Geometry check sheet. Reference: the model listing, model coordinates, mm. Face numbers are marked on the shaded views. A direction names the side the tool comes from. Round coordinates to 2 decimals unless told otherwise and drop trailing zeros. Write each loop counter-clockwise with the first axis right and the second up, starting at its lowest first coordinate (ties: lowest second). Pieces come first, ordered by that corner, then holes. Notation, with made-up numbers: (-9, 41.5) -> (29, 41.5) arc R22 ccw to (29, 48.5) -> close; hole circle Ø9 at (79, -23). An arc over 180 degrees is marked (long way). Return JSON: item names as keys, results as strings. Group by question number.
from build123d import *

# Parameters (mm, degrees)
EXTRUDE_1_DEPTH     = 3
SKETCH_2_R          = 1.6
CUT_EXTRUDE_1_DEPTH = 3


with BuildPart() as part:
    # 草图1 → 凸台-拉伸1 (new body)
    with BuildSketch(Plane.XY):
        Polygon((0, 48), (0, 0), (20, 0), (49.052558883, 16.773502692), (39.052558883, 34.094010768), (20, 23.094010768), (20, 48), align=None)
    extrude(amount=EXTRUDE_1_DEPTH)

    # 草图2 → 切除-拉伸1 (cut)
    with BuildSketch(Plane(origin=(0, 0, 0), x_dir=(-1, 0, 0), z_dir=(0, 0, -1))):
        with Locations((-42.222431864, 18.603629711)):
            Circle(SKETCH_2_R)
        with Locations((-37.222431864, 27.263883749)):
            Circle(SKETCH_2_R)
        with Locations((-26.830127019, 21.263883749)):
            Circle(SKETCH_2_R)
        with Locations((-31.830127019, 12.603629711)):
            Circle(SKETCH_2_R)
        with Locations((-16, 7)):
            Circle(SKETCH_2_R)
        with Locations((-16, 17)):
            Circle(SKETCH_2_R)
        with Locations((-4, 7)):
            Circle(SKETCH_2_R)
        with Locations((-4, 17)):
            Circle(SKETCH_2_R)
        with Locations((-16, 31)):
            Circle(SKETCH_2_R)
        with Locations((-16, 41)):
            Circle(SKETCH_2_R)
        with Locations((-4, 31)):
            Circle(SKETCH_2_R)
        with Locations((-4, 41)):
            Circle(SKETCH_2_R)
    extrude(amount=-CUT_EXTRUDE_1_DEPTH, mode=Mode.SUBTRACT)


solid = part.part
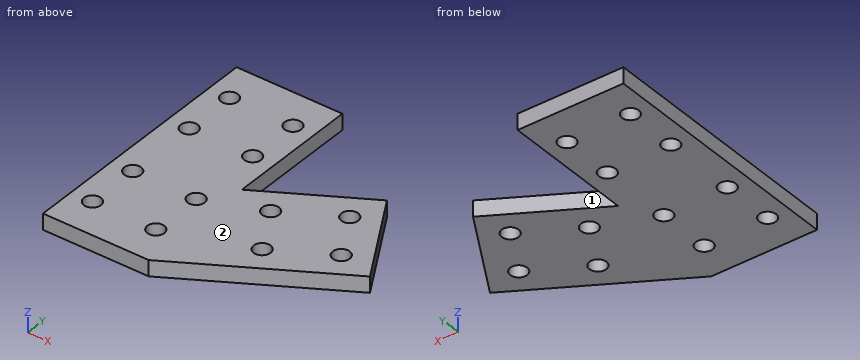
1) Sectioned sample at A-A on y = 41. Enter the section's corners in (x, z), and give its area (3 significant figures).
2) Sectioned sample at C-C on y = 31. Enter the section's corners in (x, z), and give its area (3 significant figures).
3) Sectioned sample at D-D on z = 2.05. State how many separate pieces and enclosed holes the cut face has, and give its area (3 significant figures).
4) Sectioned sample at B-B on x = 4. Enter the section's corners in (y, z).
5) Tool access check on the marked faces 1 and 2. Record the directions out of +Z, -Z, +X, -X, +Y, -Y that give a thin tool (end or side, any length) a straight path to the whole face; none if there is none.
6) Material ranges on probe 1 along Y at (x, z) = (4, 0.9); probe 2 along Y at (x, z) = (15, 2.35); probe 3 along X at (y, z) = (27.5, 1.1), recorded low to high. Write a range as [from, to].
7) Go/stop test with flat-tipped pins: P1, Ø3.5, axis at x = 16, y = 31, coming from the +Z side; P2, Ø1.5, axis at y = 25.5, z = 2, coming from the +X side. Record where each tip stops, or that it passes through.
Evaluation:
{
 "1": {"outline": "(0, 0) -> (2.4, 0) -> (2.4, 3) -> (0, 3) -> close; (5.6, 0) -> (14.4, 0) -> (14.4, 3) -> (5.6, 3) -> close; (17.6, 0) -> (20, 0) -> (20, 3) -> (17.6, 3) -> close", "area": "40.8 mm2"},
 "2": {"outline": "(0, 0) -> (2.4, 0) -> (2.4, 3) -> (0, 3) -> close; (5.6, 0) -> (14.4, 0) -> (14.4, 3) -> (5.6, 3) -> close; (17.6, 0) -> (20, 0) -> (20, 3) -> (17.6, 3) -> close; (33.69, 0) -> (40.84, 0) -> (40.84, 3) -> (33.69, 3) -> close", "area": "62.2 mm2"},
 "3": {"separate pieces": "1", "enclosed holes": "12", "area": "1,420 mm2"},
 "4": {"outline": "(0, 0) -> (5.4, 0) -> (5.4, 3) -> (0, 3) -> close; (8.6, 0) -> (15.4, 0) -> (15.4, 3) -> (8.6, 3) -> close; (18.6, 0) -> (29.4, 0) -> (29.4, 3) -> (18.6, 3) -> close; (32.6, 0) -> (39.4, 0) -> (39.4, 3) -> (32.6, 3) -> close; (42.6, 0) -> (48, 0) -> (48, 3) -> (42.6, 3) -> close"},
 "5": {"face 1": "+Z, -Z, +Y", "face 2": "+Z, +X, -X, +Y, -Y"},
 "6": {"probe 1": "y = [0, 5.4], [8.6, 15.4], [18.6, 29.4], [32.6, 39.4], [42.6, 48]", "probe 2": "y = [0, 5.75], [8.25, 15.75], [18.25, 29.75], [32.25, 39.75], [42.25, 48]", "probe 3": "x = [0, 20], [27.63, 35.64], [38.8, 42.86]"},
 "7": {"P1": "stops at z = 3", "P2": "stops at x = 44.45"}
}
